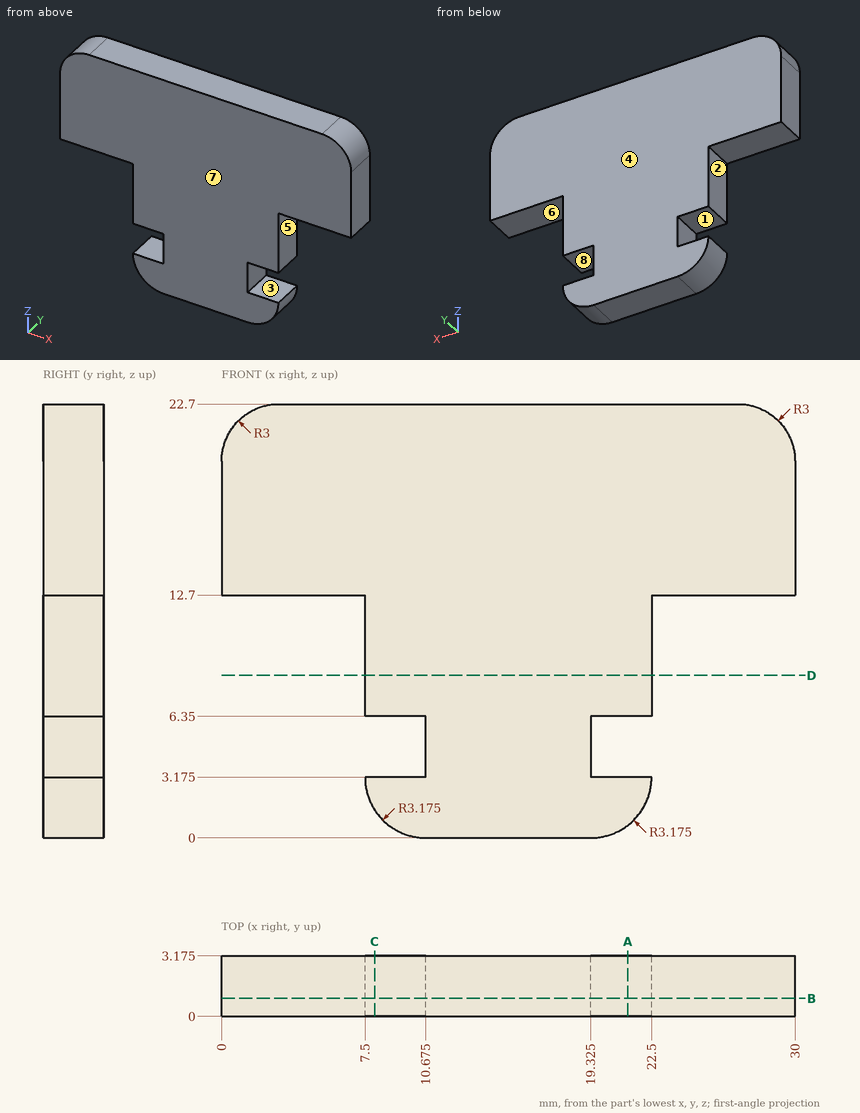
For this review, use the dimensioned drawing (mm, ordinates from the lowest corner) and the shaded views. A direction names the side the tool comes from. Give positions to 0.01 mm unless a question says otherwise; leave off trailing zeros. Order: outer loops, then holes, each group sorted by start corner. A loop starts at its lowest first (then second) coordinate and runs counter-clockwise, first axis right, second up. Notation, with made-up numbers: (8, 52) - (40, 52) arc R7 ccw to (40, 59) - close; hole circle Ø3 at (36.5, 16). An arc over 180 degrees is marked (long way). Use CSV: the item, a comma, the result in double quotes. Start each with the question number.
Q1. The part is to be moulded in two halves that separate along Z. For the marked faces 6, 7 and 8, say which applies: +Z half, -Z half, draft (parallel to the pull), parting line (faces both ways), or undercut.
Q2. We need section A-A, the plane x = 21.25. Write out the cut boundary in (y, z) (3 decimals).
Q3. We need section B-B, the plane y = 0.95. Write out the cut boundary in (x, z) (3 decimals), and give its area (3 significant figures).
Q4. We need section C-C, the plane x = 8. Write out the cut boundary in (y, z) (3 decimals), and give its area (3 significant figures).
Q5. To check wall thickness, follow line 1 along Z through (x, y) = (23.5, 2.75); line 2 along X through (y, z) = (2.15, 4) (3 decimals); line 3 along Z through (x, y) = (9, 2.45) (3 decimals). State the ranges of each line that lie inside material, in increasing order. Write a range as [from, to].
Q6. Tool access review of the marked faces 1, 2, 3, 4 and 5: name each direction out of +Z, -Z, +X, -X, +Y, -Y from which nothing blocks a thin tool from reaching the whole face with its end or side.
Q7. We need section D-D, the plane z = 8.5. Write out the cut boundary in (x, y) (3 decimals).
Q8. Clearance check with flat-ended pins moving along their axes: pin 1 Ø1.6 at (y, z) = (1, 5) entering from -X (3 decimals); pin 2 Ø1 at (x, y) = (25, 1.5) entering from -Z; pin 3 Ø1.6 at (y, z) = (1, 10) entering from -X. State where each tip first meets the part, or that it passes through.
Outcome:
1,face 6,"-Z half"
1,face 7,"draft"
1,face 8,"undercut"
2,outline,"(0, 0.65) - (3.175, 0.65) - (3.175, 3.175) - (0, 3.175) - close; (0, 6.35) - (3.175, 6.35) - (3.175, 22.7) - (0, 22.7) - close"
3,outline,"(0, 12.7) - (7.5, 12.7) - (7.5, 6.35) - (10.675, 6.35) - (10.675, 3.175) - (7.5, 3.175) arc R3.175 ccw to (10.675, 0) - (19.325, 0) arc R3.175 ccw to (22.5, 3.175) - (19.325, 3.175) - (19.325, 6.35) - (22.5, 6.35) - (22.5, 12.7) - (30, 12.7) - (30, 19.7) arc R3 ccw to (27, 22.7) - (3, 22.7) arc R3 ccw to (0, 19.7) - close"
3,area,"462 mm^2"
4,outline,"(0, 1.465) - (3.175, 1.465) - (3.175, 3.175) - (0, 3.175) - close; (0, 6.35) - (3.175, 6.35) - (3.175, 22.7) - (0, 22.7) - close"
4,area,"57.3 mm^2"
5,line 1,"z = [12.7, 22.7]"
5,line 2,"x = [10.675, 19.325]"
5,line 3,"z = [0.478, 3.175], [6.35, 22.7]"
6,face 1,"-X, +Y, -Y"
6,face 2,"-Z, -X, +Y, -Y"
6,face 3,"+X, +Y, -Y"
6,face 4,"+Z, -Z, +X, -X, +Y"
6,face 5,"-Z, +X, +Y, -Y"
7,outline,"(7.5, 0) - (22.5, 0) - (22.5, 3.175) - (7.5, 3.175) - close"
8,pin 1,"stops at x = 10.675"
8,pin 2,"stops at z = 12.7"
8,pin 3,"stops at x = 7.5"
